from build123d import *

# Parameters (mm, degrees)
CHAMFER1_SIZE           = 0.762
CUT_EXTRUDE1_DEPTH      = 14.919
CUT_EXTRUDE1_DEPTH_BACK = 14.919
HOLE1_D                 = 5.0038
HOLE1_DEPTH             = 4.064
CIRPATTERN1_COUNT       = 4
SKETCH6_W               = 6.35
SKETCH6_H               = 2.019
CUT_EXTRUDE2_DEPTH      = 14.919
CUT_EXTRUDE2_DEPTH_BACK = 14.919


with BuildPart() as part:
    # Sketch1 → Revolve1 (revolve)
    with BuildSketch(Plane(origin=(0, 0, 0), x_dir=(-1, 0, 0), z_dir=(0, 0, -1)), mode=Mode.PRIVATE) as revolve1_sk:
        with BuildLine():
            Line((-59.2328, 5.707922533), (-59.2328, 0))
            Line((-59.2328, 0), (0, 0))
            Line((0, 0), (0, 12.319))
            Line((0, 12.319), (-12.7, 12.319))
            Line((-12.7, 12.319), (-14.3, 13.919))
            Line((-14.3, 13.919), (-46.5838, 13.919))
            Line((-46.5838, 13.919), (-48.1838, 12.319))
            Line((-48.1838, 12.319), (-49.1998, 12.319))
            Line((-49.1998, 12.319), (-49.1998, 6.3373))
            Line((-49.1998, 6.3373), (-52.9082, 6.3373))
            Line((-52.9082, 6.3373), (-53.6702, 6.096))
            Line((-53.6702, 6.096), (-58.2168, 6.096))
            ThreePointArc((-58.2168, 6.096), (-58.760596865, 5.995678675), (-59.2328, 5.707922533))
        make_face()
    revolve(revolve1_sk.sketch.rotate(Axis((59.2328, 0, 0), (-1, 0, 0)), 270), axis=Axis((59.2328, 0, 0), (-1, 0, 0)))  # turned: the seam where the file's is

    # Sketch2 → Cut-Revolve1 (revolve, cut)
    with BuildSketch(Plane(origin=(0, 0, 0), x_dir=(-1, 0, 0), z_dir=(0, 0, -1)), mode=Mode.PRIVATE) as cut_revolve1_sk:
        Polygon((-10.5664, 0), (-10.5664, 4.4196), (-0.6604, 4.4196), (-0.127, 4.953), (0, 4.953), (0, 0), align=None)
    revolve(cut_revolve1_sk.sketch.rotate(Axis((33.143328407, 0, 0), (-1, 0, 0)), 270), axis=Axis((33.143328407, 0, 0), (-1, 0, 0)), mode=Mode.SUBTRACT)  # turned: the seam where the file's is

    # Sketch3 → Cut-Revolve2 (revolve, cut)
    with BuildSketch(Plane(origin=(0, 0, 0), x_dir=(-1, 0, 0), z_dir=(0, 0, -1)), mode=Mode.PRIVATE) as cut_revolve2_sk:
        Polygon((-59.2328, 2.5146), (-59.2328, 0), (-48.0568, 0), (-49.567724113, 2.5146), align=None)
    revolve(cut_revolve2_sk.sketch.rotate(Axis((66.313858967, 0, 0), (-1, 0, 0)), 270), axis=Axis((66.313858967, 0, 0), (-1, 0, 0)), mode=Mode.SUBTRACT)  # turned: the seam where the file's is

    # Chamfer1
    chamfer1_edges = [part.edges().sort_by_distance(p)[0] for p in [
        (0, 0, -12.319),
    ]]
    chamfer(chamfer1_edges, length=CHAMFER1_SIZE)

    # Sketch4 → Cut-Extrude1 (cut, two sides)
    with BuildSketch(Plane(origin=(0, 0, 0), x_dir=(1, 0, 0), z_dir=(0, 1, 0))) as cut_extrude1_sk:
        Polygon((53.8226, 6.096), (54.4576, 5.461), (59.2328, 5.461), (59.2328, 6.096), align=None)
        Polygon((59.2328, -6.096), (53.8226, -6.096), (54.4576, -5.461), (59.2328, -5.461), align=None)
    extrude(amount=CUT_EXTRUDE1_DEPTH, mode=Mode.SUBTRACT)
    extrude(cut_extrude1_sk.sketch, amount=-CUT_EXTRUDE1_DEPTH_BACK, mode=Mode.SUBTRACT)

    # Hole1
    with Locations(Plane(origin=(5.588, 12.319, 0), x_dir=(0, 0, 1), z_dir=(0, 1, 0))):
        with Locations((0, 0)):
            hole1 = Hole(HOLE1_D / 2, depth=HOLE1_DEPTH)

    # CirPattern1: Hole1 ×4 about axis
    cirpattern1_axis = Axis((0, 0, 0), (1, 0, 0))
    for i in range(1, CIRPATTERN1_COUNT):
        add(hole1.rotate(cirpattern1_axis, i * 360 / CIRPATTERN1_COUNT), mode=Mode.SUBTRACT)

    # Sketch6 → Cut-Extrude2 (cut, two sides)
    with BuildSketch(Plane(origin=(0, 0, 0), x_dir=(1, 0, 0), z_dir=(0, 1, 0))) as cut_extrude2_sk:
        with Locations((46.0248, 12.9095)):
            Rectangle(SKETCH6_W, SKETCH6_H)
        with Locations((46.0248, -12.9095)):
            Rectangle(SKETCH6_W, SKETCH6_H)
    extrude(amount=CUT_EXTRUDE2_DEPTH, mode=Mode.SUBTRACT)
    extrude(cut_extrude2_sk.sketch, amount=-CUT_EXTRUDE2_DEPTH_BACK, mode=Mode.SUBTRACT)


solid = part.part
For this review, take the finished solid that the model builds, in its own axes (mm). A direction names the side the tool comes from. Give positions to 0.01 mm unless a question says otherwise; leave off trailing zeros. Loops run counter-clockwise (first coordinate to the right, second up) from the corner with the lowest first, then second, coordinate; pieces in that order, holes last.
Item 1: For line 1 along X through (y, z) = (-9.2, 0); line 2 along Y through (x, z) = (57.25, 0); line 3 along Y through (x, z) = (0.1, 0), list the stretches that pass through material, from the lowest coordinate up.
Item 2: Tool access review of faces 1 (the flat face through (10.566, 0, 0)), 2 (the flat face through (57, 0, 5.461)), 3 (the flat face through (49.2, -5, 5)), 4 (the cylindrical face through (4.6, 2.3, 10.3)), 5 (the flat face through (42.85, 0, -13)): name each direction out of +Z, -Z, +X, -X, +Y, -Y from which nothing blocks a thin tool from reaching the whole face with its end or side.
Item 3: Draft analysis for pull direction Z (two halves, no side actions). For faces 6 (the cylindrical face through (4.6, -2.3, -10.3)), 7 (the conical face through (48.32, -0.43, -0.09)), 8 (the flat face through (6, 0, -8.255)), 9 (the cylindrical face through (30.668, 0.612, -13.906)), state which applies: +Z half, -Z half, draft (parallel to the pull), parting line (faces both ways), or undercut.
Item 4: Insertion check: pin 1 (1.6 mm diameter, centred on y = 2, z = -12.5, fed in from +X); pin 2 (3 mm diameter, centred on x = 5.588, y = 0, fed in from -Z) (3 decimals); pin 3 (1 mm diameter, centred on x = 14.5, z = -3, fed in from +Y); pin 4 (1.5 mm diameter, centred on y = 5, z = -3.5, fed in from +X). Each pin has a flat end and moves straight along its axis. Give the tip position at first contact, or say it passes through.
Item 5: Take a section at B-B, the plane x = 21. State the section outline as (y, z) points.
Item 6: Take a section at A-A, the plane x = 50.5. State the section outline as (y, z) points, and give its area (3 significant figures).
Calculated:
1. line 1: x = 0 to 3.09, 8.09 to 49.2
1. line 2: y = -6.1 to -2.51, 2.51 to 6.1
1. line 3: y = -11.66 to -4.95, 4.95 to 11.66
2. face 1: -X
2. face 2: +Z, +X, +Y, -Y
2. face 3: +X
2. face 4: +Z
2. face 5: -Z, +X, +Y, -Y
3. face 6: draft
3. face 7: undercut
3. face 8: -Z half
3. face 9: parting line
4. pin 1: stops at x = 49.2
4. pin 2: stops at z = -8.255
4. pin 3: stops at y = 13.69
4. pin 4: stops at x = 59.23
5. outline: circle Ø27.84 at (0, 0)
6. outline: circle Ø12.67 at (0, 0); hole circle Ø5.03 at (0, 0)
6. area: 106 mm2
